from build123d import *

# Parameters (mm, degrees)
PAD_DEPTH = 4
FILLET_R  = 1


with BuildPart() as part:
    # Sketch → Pad (new body)
    with BuildSketch(Plane.XY):
        Polygon((0, 0), (53, 53), (106, 0), align=None)
    extrude(amount=PAD_DEPTH)

    # Fillet
    fillet_edges = [part.edges().sort_by_distance(p)[0] for p in [
        (0, 0, 2),
        (53, 53, 2),
        (26.5, 26.5, 0),
        (26.5, 26.5, 4),
        (106, 0, 2),
        (79.5, 26.5, 0),
        (79.5, 26.5, 4),
        (53, 0, 0),
        (53, 0, 4),
    ]]
    fillet(fillet_edges, radius=FILLET_R)


solid = part.part
Input: part model. Units: mm. Frame: model coordinates. Give positions to 0.01 mm unless a question says otherwise; leave off trailing zeros. Write each loop counter-clockwise with the first axis right and the second up, starting at its lowest first coordinate (ties: lowest second). Pieces come first, ordered by that corner, then holes. Notation, with made-up numbers: (-12.5, 63.5) -> (6.5, 63.5) arc R27 cw to (6.5, 97.5) -> close; hole circle Ø7 at (51.25, -33). An arc over 180 degrees is marked (long way). Use one line per item in the form item = value. Start each with the question number.
1) Pin query (flat end, axial travel): pin 1 (1.5 mm diameter, centred on x = 79.5, y = 14, fed in from -Z); pin 2 (2 mm diameter, centred on y = 42.5, z = 3.5, fed in from -X). Return the tip coordinate at first contact, or that it passes through.
2) Ray query, probe 1 along X at (y, z) = (11.5, 1.95); probe 2 along X at (y, z) = (48, 3.35); probe 3 along Y at (x, z) = (35, 3.7). Return the intervals inside material, ascending. Write a range as from..to.
3) Section query A-A on z = 1.8. Return the cut outline in (x, y).
Outcome:
q1.pin_1 = 0
q1.pin_2 = 41.57
q2.probe_1 = 11.5..94.5
q2.probe_2 = 48.09..57.91
q2.probe_3 = 0.29..34.6
q3.outline = (1.71, 1.71) arc R1 ccw to (2.41, 0) -> (103.59, 0) arc R1 ccw to (104.29, 1.71) -> (53.71, 52.29) arc R1 ccw to (52.29, 52.29) -> close
